```python
from build123d import *

# Parameters (mm, degrees)
SKETCH1_R           = 1
BOSS_EXTRUDE1_DEPTH = 9
CHAMFER1_SIZE       = 2
SKETCH5_R           = 1.411016717
CUT_EXTRUDE4_DEPTH  = 32.657609573
CUT_EXTRUDE5_DEPTH  = 32.657609573
SKETCH7_R           = 3
CUT_EXTRUDE6_DEPTH  = 5


with BuildPart() as part:
    # Sketch1 → Boss-Extrude1 (new body)
    with BuildSketch(Plane(origin=(0, 0, 0), x_dir=(0, 0, -1), z_dir=(1, 0, 0))):
        Polygon((-7.5, 0), (7.5, 0), (7.5, 15.76), (4.103828097, 28.939458123), (-9.149426619, 17.160897736), (-7.5, 10.76), align=None)
        with Locations((2.957491833, 21.231429279)):
            Circle(SKETCH1_R, mode=Mode.SUBTRACT)
        with Locations((-1.901052893, 16.913496539)):
            Circle(SKETCH1_R, mode=Mode.SUBTRACT)
    extrude(amount=BOSS_EXTRUDE1_DEPTH)

    # Chamfer1
    chamfer1_edges = [part.edges().sort_by_distance(p)[0] for p in [
        (4.5, 0, -7.5),
        (9, 0, 0),
    ]]
    chamfer(chamfer1_edges, length=CHAMFER1_SIZE)

    # Sketch5 → Cut-Extrude4 (cut, through all)
    with BuildSketch(Plane(origin=(9, 0, 0), x_dir=(0, 0, -1), z_dir=(1, 0, 0))):
        with Locations((3.500000028, 6.380001803)):
            Circle(SKETCH5_R)
        with Locations((-3.5, 6.380001848)):
            Circle(SKETCH5_R)
    extrude(amount=-CUT_EXTRUDE4_DEPTH, mode=Mode.SUBTRACT)

    # Sketch6 → Cut-Extrude5 (cut, through all)
    with BuildSketch(Plane(origin=(9, 0, 0), x_dir=(0, 0, -1), z_dir=(1, 0, 0))):
        Polygon((1.990530631, 27.061308011), (5.648400148, 22.945467464), (4.103828097, 28.939458123), align=None)
    extrude(amount=-CUT_EXTRUDE5_DEPTH, mode=Mode.SUBTRACT)

    # Sketch7 → Cut-Extrude6 (cut)
    with BuildSketch(Plane(origin=(9, 0, 0), x_dir=(0, 0, -1), z_dir=(1, 0, 0))):
        with Locations((3.500000028, 6.380001803)):
            Circle(SKETCH7_R)
        with Locations((-3.5, 6.380001848)):
            Circle(SKETCH7_R)
    extrude(amount=-CUT_EXTRUDE6_DEPTH, mode=Mode.SUBTRACT)


solid = part.part
```
Could you check a few things on this model? Use its own coordinates, in mm. A direction names the side the tool comes from. Coordinates: 2 decimals unless noted, no trailing zeros. Write each loop counter-clockwise with the first axis right and the second up, starting at its lowest first coordinate (ties: lowest second). Pieces come first, ordered by that corner, then holes. Notation, with made-up numbers: (24.25, 28.25) -> (82.25, 28.25) arc R13 ccw to (82.25, 46.25) -> close; hole circle Ø3 at (25.25, 72). An arc over 180 degrees is marked (long way). One line per question, with ' | ' between items. Start each with the question number.
1. Please list where these lines run through material, in increasing order: line 1 along Z through (x, y) = (8.75, 6.5); line 2 along Y through (x, z) = (6.9, -3.5); line 3 along Y through (x, z) = (2.1, -3.5).
2. If we section it at C-C (z = 3.5): Please give me the cut outline in (x, y), and give its area (3 significant figures).
3. Will these pins go through, and if not, where does the flat tip stop? P1, Ø5, axis at x = 5, y = 21, coming from the -Z side; P2, Ø3.5, axis at y = 6.38, z = -3.5, coming from the +X side; P3, Ø2, axis at x = 3, y = 21.5, coming from the +Z side.
4. If we section it at A-A (y = 20.75): Please give me the cut outline in (x, z).
5. If we section it at D-D (y = 4): Please give me the cut outline in (x, z).
6. If we section it at B-B (z = -3.5): Please give me the cut outline in (x, y).
7. Thinking about a two-plate mould opening in Y: for faces 4 (the face through (4.437, 19.302, -6.587)), 5 (the face through (4.437, 14.005, 8.336)), 6 (the face through (4, 7, 2)), 7 (the face through (6.54, 7.28, -6.36)), which applies, pulls with the +Y half, pulls with the -Y half, needs draft (parallel to the pull), parting line crosses it, or undercut?
8. For faces 1 (the face through (4.437, 21.907, -2.22)), 2 (the face through (6.54, 3.45, 4.15)), 3 (the face through (4, 5, 7.5)), which set-ups out of +Z, -Z, +X, -X, +Y, -Y let a thin tool reach every point of the face, with its end or its side?
Return value:
1) line 1: z = -7.5 to -6.5, -0.5 to 0.5, 6.5 to 7.5 | line 2: y = 0 to 3.38, 9.38 to 20.39, 22.07 to 25.36 | line 3: y = 0 to 4.97, 7.79 to 20.39, 22.07 to 25.36
2) outline: (0, 0) -> (7, 0) -> (9, 2) -> (9, 3.38) -> (4, 3.38) -> (4, 4.97) -> (0, 4.97) -> close; (0, 7.79) -> (4, 7.79) -> (4, 9.38) -> (9, 9.38) -> (9, 22.18) -> (0, 22.18) -> close | area: 156 mm²
3) P1: stops at z = -6.79 | P2: stops at x = 4 | P3: stops at z = 5.39
4) outline: (0, -6.21) -> (9, -6.21) -> (9, -3.83) -> (0, -3.83) -> close; (0, -2.08) -> (9, -2.08) -> (9, 5.11) -> (0, 5.11) -> close
5) outline: (0, -7.5) -> (9, -7.5) -> (9, -5.33) -> (4, -5.33) -> (4, -1.67) -> (9, -1.67) -> (9, 1.67) -> (4, 1.67) -> (4, 5.33) -> (9, 5.33) -> (9, 7.5) -> (0, 7.5) -> close
6) outline: (0, 0) -> (7, 0) -> (9, 2) -> (9, 3.38) -> (4, 3.38) -> (4, 4.97) -> (0, 4.97) -> close; (0, 7.79) -> (4, 7.79) -> (4, 9.38) -> (9, 9.38) -> (9, 20.39) -> (0, 20.39) -> close; (0, 22.07) -> (9, 22.07) -> (9, 25.36) -> (0, 25.36) -> close
7) face 4: pulls with the +Y half | face 5: pulls with the -Y half | face 6: undercut | face 7: undercut
8) face 1: +X, -X | face 2: +X | face 3: +Z, +X, -X, -Y
